Could you check a few things on this model? Use its own coordinates, in mm. Face numbers are marked on the shaded views. A direction names the side the tool comes from. Give positions to 0.01 mm unless a question says otherwise; leave off trailing zeros. Write each loop counter-clockwise with the first axis right and the second up, starting at its lowest first coordinate (ties: lowest second). Pieces come first, ordered by that corner, then holes. Notation, with made-up numbers: M -17.75,85.25 L 36.25,85.25 A19 cw 36.25,96.25 Z; hole C 22,-39.5 d7. An arc over 180 degrees is marked long. Use one line per item in the form item = value.
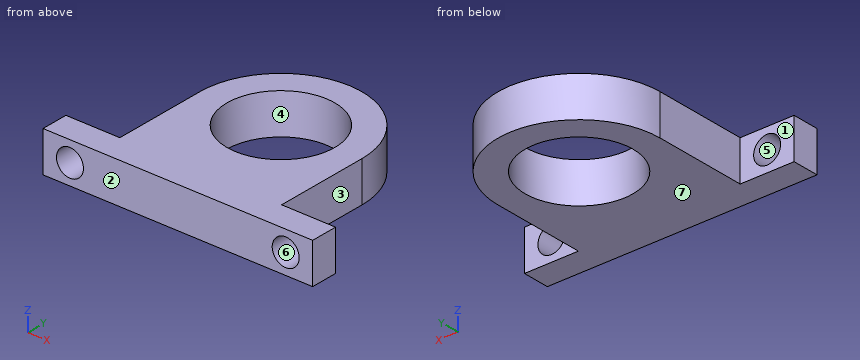
from build123d import *

# Parameters (mm, degrees)
SKETCH1_W           = 20
SKETCH1_H           = 2
BOSS_EXTRUDE1_DEPTH = 3
SKETCH2_R           = 1
CUT_EXTRUDE1_DEPTH  = 16


with BuildPart() as part:
    # Sketch1 → Boss-Extrude1 (new body)
    with BuildSketch(Plane.XY):
        with Locations((0, 1)):
            Rectangle(SKETCH1_W, SKETCH1_H)
        with BuildLine():
            Line((-6, 9), (-6, 2))
            Line((-6, 2), (6, 2))
            Line((6, 2), (6, 9))
            ThreePointArc((6, 9), (0, 3), (-6, 9))
        make_face()
        with BuildLine():
            ThreePointArc((6, 9), (0, 15), (-6, 9))
            Line((-6, 9), (-4, 9))
            ThreePointArc((-4, 9), (0, 13), (4, 9))
            Line((4, 9), (6, 9))
        make_face()
        with BuildLine():
            Line((-4, 9), (-6, 9))
            ThreePointArc((-6, 9), (0, 3), (6, 9))
            Line((6, 9), (4, 9))
            ThreePointArc((4, 9), (0, 5), (-4, 9))
        make_face()
    extrude(amount=BOSS_EXTRUDE1_DEPTH)

    # Sketch2 → Cut-Extrude1 (cut, through all)
    with BuildSketch(Plane(origin=(0, 0, 0), x_dir=(1, 0, 0), z_dir=(0, 1, 0))):
        with Locations((-8, -1.5)):
            Circle(SKETCH2_R)
        with Locations((8, -1.5)):
            Circle(SKETCH2_R)
    extrude(amount=CUT_EXTRUDE1_DEPTH, mode=Mode.SUBTRACT)


solid = part.part
1) I want a section at D-D, the plane x = 4.5. Please give me the cut outline in (y, z), plus the area to 3 significant figures.
Checked values:
outline = M 0,0 L 12.97,0 L 12.97,3 L 0,3 Z
area = 38.9 mm2
2) Thinking about a two-plate mould opening in Z: for the marked faces 4, 5, 6 and 7, which applies, released by +Z, released by -Z, zero draft, split by the parting line, or undercut?
Checked values:
face_4 = zero draft
face_5 = undercut
face_6 = undercut
face_7 = released by -Z
3) For pin 1 Ø0.9 at (x, z) = (9, 1.5) entering from +Y, with a flat end and sliding along its axis, tell me the tip position at first contact or that it passes through.
Checked values:
pin_1 = 2
4) For the marked faces 1, 2 and 3, which set-ups out of +Z, -Z, +X, -X, +Y, -Y let a thin tool reach every point of the face, with its end or its side?
Checked values:
face_1 = +Z, -Z, -X, +Y
face_2 = +Z, -Z, +X, -X, -Y
face_3 = +Z, -Z, +X, +Y
5) If I drill on L1, parallel to X at y = 1, z = 1.5; L2, parallel to Y at x = 0, z = 1; L3, parallel to Z at x = -8, y = 1.1, over which ranges is the centre line in solid material (lowest first)?
Checked values:
L1 = -10 to -9, -7 to 7, 9 to 10
L2 = 0 to 5, 13 to 15
L3 = 0 to 0.5, 2.5 to 3
6) I want a section at C-C, the plane y = 7. Please give me the cut outline in (x, z), plus the area to 3 significant figures.
Checked values:
outline = M -6,0 L -3.46,0 L -3.46,3 L -6,3 Z; M 3.46,0 L 6,0 L 6,3 L 3.46,3 Z
area = 15.2 mm2
7) I want a section at B-B, the plane x = -8. Please give me the cut outline in (y, z), plus the area to 3 significant figures.
Checked values:
outline = M 0,0 L 2,0 L 2,0.5 L 0,0.5 Z; M 0,2.5 L 2,2.5 L 2,3 L 0,3 Z
area = 2.00 mm2
8) I want a section at A-A, the plane z = 1.5. Please give me the cut outline in (x, y).
Checked values:
outline = M -10,0 L -9,0 L -9,2 L -10,2 Z; M -7,0 L 7,0 L 7,2 L 6,2 L 6,9 A6 ccw -6,9 L -6,2 L -7,2 Z; M 9,0 L 10,0 L 10,2 L 9,2 Z; hole C 0,9 d8
